Autodesk Inventor part; units mm, degrees
ref_plane "IP_1_XY" through (4.5, 0, 0) normal (1, 0, 0) x (0, 0, -1)
ref_plane "IP_1_YZ" through (4.5, 0, 0) normal (0, 0, -1) x (0, 1, 0)
ref_plane "IP_1_ZX" through (4.5, 0, 0) normal (0, 1, 0) x (1, 0, 0)
sketch "Sketch_1" plane through (0, 0, 0) normal (0, 0, 1) x (1, 0, 0)
  line L0 (8.3, 0) -> (0.7, 0)
  line L1 (0.7, 3.875) -> (8.3, 3.875)
  line L2 (8.3, 3.875) -> (8.3, 4.625)
  line L3 (8.3, 4.625) -> (0.7, 4.625)
  line L4 (0.7, 4.625) -> (0.7, 3.875)
revolve "Revolution1" add sketch "Sketch_1" angle 360 about axis through (8.3, 0, 0) along (1, 0, 0)
sketch "Sketch_2" plane through (0, 0, 0) normal (0, 0, 1) x (1, 0, 0)
  line L0 (7, 4.25) -> (2, 4.25)
  line L1 (2, 4.25) -> (2, 5)
  line L2 (2, 5) -> (7, 5)
  line L3 (7, 5) -> (7, 4.25)
  line L4 (7, 4.25) -> (2, 4.25)
revolve "Revolution2" cut sketch "Sketch_2" angle 360 about axis through (7, 4.25, 0) along (1, 0, 0)
pattern_circular "Circular Pattern1" count 10 over 360 about axis through (4.5, 0, 0) along (1, 0, 0) of "Revolution2"
ref_plane "IP_1_XY" through (4.5, 0, 0) normal (1, 0, 0) x (0, 0, -1)
ref_plane "IP_1_YZ" through (4.5, 0, 0) normal (0, 0, -1) x (0, 1, 0)
ref_plane "IP_1_ZX" through (4.5, 0, 0) normal (0, 1, 0) x (1, 0, 0)
ref_plane "IP_3_1_XY" through (4.5, 4.25, 0) normal (1, 0, 0) x (0, 0, -1)
ref_plane "IP_3_1_YZ" through (4.5, 4.25, 0) normal (0, 0, -1) x (0, 1, 0)
ref_plane "IP_3_1_ZX" through (4.5, 4.25, 0) normal (0, 1, 0) x (1, 0, 0)
ref_plane "IP_3_10_XY" through (4.5, 3.4383, -2.4981) normal (1, 0, 0) x (0, 0, -1)
ref_plane "IP_3_10_YZ" through (4.5, 3.4383, -2.4981) normal (0, 0, -1) x (0, 1, 0)
ref_plane "IP_3_10_ZX" through (4.5, 3.4383, -2.4981) normal (0, 1, 0) x (1, 0, 0)
ref_plane "IP_3_2_XY" through (4.5, 3.4383, 2.4981) normal (1, 0, 0) x (0, 0, -1)
ref_plane "IP_3_2_YZ" through (4.5, 3.4383, 2.4981) normal (0, 0, -1) x (0, 1, 0)
ref_plane "IP_3_2_ZX" through (4.5, 3.4383, 2.4981) normal (0, 1, 0) x (1, 0, 0)
ref_plane "IP_3_3_XY" through (4.5, 1.3133, 4.042) normal (1, 0, 0) x (0, 0, -1)
ref_plane "IP_3_3_YZ" through (4.5, 1.3133, 4.042) normal (0, 0, -1) x (0, 1, 0)
ref_plane "IP_3_3_ZX" through (4.5, 1.3133, 4.042) normal (0, 1, 0) x (1, 0, 0)
ref_plane "IP_3_4_XY" through (4.5, -1.3133, 4.042) normal (1, 0, 0) x (0, 0, -1)
ref_plane "IP_3_4_YZ" through (4.5, -1.3133, 4.042) normal (0, 0, -1) x (0, 1, 0)
ref_plane "IP_3_4_ZX" through (4.5, -1.3133, 4.042) normal (0, 1, 0) x (1, 0, 0)
ref_plane "IP_3_5_XY" through (4.5, -3.4383, 2.4981) normal (1, 0, 0) x (0, 0, -1)
ref_plane "IP_3_5_YZ" through (4.5, -3.4383, 2.4981) normal (0, 0, -1) x (0, 1, 0)
ref_plane "IP_3_5_ZX" through (4.5, -3.4383, 2.4981) normal (0, 1, 0) x (1, 0, 0)
ref_plane "IP_3_6_XY" through (4.5, -4.25, 0) normal (1, 0, 0) x (0, 0, -1)
ref_plane "IP_3_6_YZ" through (4.5, -4.25, 0) normal (0, 0, -1) x (0, 1, 0)
ref_plane "IP_3_6_ZX" through (4.5, -4.25, 0) normal (0, 1, 0) x (1, 0, 0)
ref_plane "IP_3_7_XY" through (4.5, -3.4383, -2.4981) normal (1, 0, 0) x (0, 0, -1)
ref_plane "IP_3_7_YZ" through (4.5, -3.4383, -2.4981) normal (0, 0, -1) x (0, 1, 0)
ref_plane "IP_3_7_ZX" through (4.5, -3.4383, -2.4981) normal (0, 1, 0) x (1, 0, 0)
ref_plane "IP_3_8_XY" through (4.5, -1.3133, -4.042) normal (1, 0, 0) x (0, 0, -1)
ref_plane "IP_3_8_YZ" through (4.5, -1.3133, -4.042) normal (0, 0, -1) x (0, 1, 0)
ref_plane "IP_3_8_ZX" through (4.5, -1.3133, -4.042) normal (0, 1, 0) x (1, 0, 0)
ref_plane "IP_3_9_XY" through (4.5, 1.3133, -4.042) normal (1, 0, 0) x (0, 0, -1)
ref_plane "IP_3_9_YZ" through (4.5, 1.3133, -4.042) normal (0, 0, -1) x (0, 1, 0)
ref_plane "IP_3_9_ZX" through (4.5, 1.3133, -4.042) normal (0, 1, 0) x (1, 0, 0)
properties part number "HK0709FMCA" material "Steel"
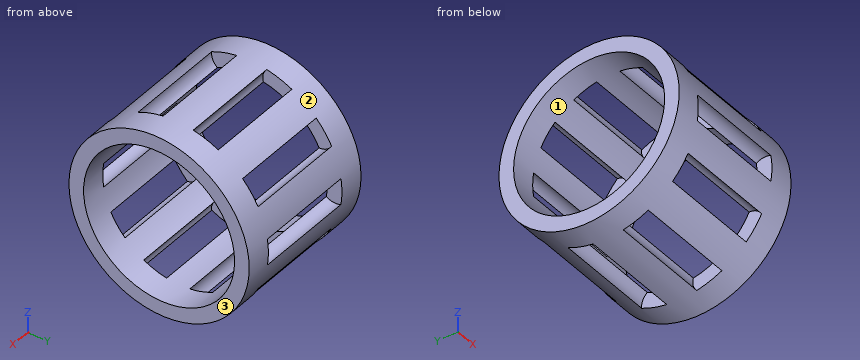
Verification items for the finished model (mm, model axes). Face numbers are marked on the shaded views. Give positions to 0.01 mm unless a question says otherwise; leave off trailing zeros. Loops run counter-clockwise (first coordinate to the right, second up) from the corner with the lowest first, then second, coordinate; pieces in that order, holes last.
1. Thickness scan on line 1 (Z direction, x = 5.5, y = 0) (3 decimals); line 2 (X direction, y = 4, z = -0.5); line 3 (Y direction, x = 3.5, z = -1). Record the ranges inside material, lowest first.
2. Section check C-C, the plane y = -1. Enter the section's corners in (x, z).
3. Go/stop test with flat-tipped pins: pin 1 Ø4 at (x, z) = (4.5, 3.5) entering from -Y (3 decimals); pin 2 Ø1.5 at (x, y) = (2, -1) entering from +Z; pin 3 Ø3 at (x, z) = (5, 2) entering from -Y. Record where each tip stops, or that it passes through.
4. Section check B-B, the plane y = 0. Enter the section's corners in (x, z) (3 decimals), then the cut area to 3 significant figures.
5. Mould release check, pull along Y, two halves, no side actions. Record for the marked faces 1, 2 and 3: released by +Y, released by -Y, zero draft, split by the parting line, or undercut.
6. Section check D-D, the plane z = -1.25. Enter the section's corners in (x, y), then the cut area to 3 significant figures.
7. Section check A-A, the plane z = 0. Enter the section's corners in (x, y) (3 decimals), then the cut area to 3 significant figures.
Geometry says:
1. line 1: z = -4.625 to -3.875, 3.875 to 4.625
1. line 2: x = 0.7 to 2, 7 to 8.3
1. line 3: y = -4.52 to -3.74, 3.74 to 4.52
2. outline: (0.7, -4.52) - (2, -4.52) - (2, -3.74) - (0.7, -3.74) - close; (0.7, 3.74) - (2, 3.74) - (2, 4.52) - (0.7, 4.52) - close; (7, -4.52) - (8.3, -4.52) - (8.3, -3.74) - (7, -3.74) - close; (7, 3.74) - (8.3, 3.74) - (8.3, 4.52) - (7, 4.52) - close
3. pin 1: stops at y = -4.375
3. pin 2: stops at z = 4.62
3. pin 3: stops at y = -4.58
4. outline: (0.7, -4.625) - (8.3, -4.625) - (8.3, -3.875) - (0.7, -3.875) - close; (0.7, 3.875) - (8.3, 3.875) - (8.3, 4.625) - (0.7, 4.625) - close
4. area: 11.4 mm2
5. face 1: undercut
5. face 2: split by the parting line
5. face 3: zero draft
6. outline: (0.7, -4.45) - (8.3, -4.45) - (8.3, -3.67) - (0.7, -3.67) - close; (0.7, 3.67) - (8.3, 3.67) - (8.3, 4.45) - (0.7, 4.45) - close
6. area: 11.9 mm2
7. outline: (0.7, -4.625) - (2, -4.625) - (2, -3.875) - (0.7, -3.875) - close; (0.7, 3.875) - (2, 3.875) - (2, 4.625) - (0.7, 4.625) - close; (7, -4.625) - (8.3, -4.625) - (8.3, -3.875) - (7, -3.875) - close; (7, 3.875) - (8.3, 3.875) - (8.3, 4.625) - (7, 4.625) - close
7. area: 3.90 mm2
